CAD build for the part. Positions are in the model's coordinates, mm. Face numbers are marked on the shaded views. Give positions to 0.01 mm unless a question says otherwise; leave off trailing zeros. Write each loop counter-clockwise with the first axis right and the second up, starting at its lowest first coordinate (ties: lowest second). Pieces come first, ordered by that corner, then holes. Notation, with made-up numbers: (-30.5, -15.5) - (-0.5, -15.5) arc R27 cw to (-0.5, 2.5) - close; hole circle Ø2 at (31.25, 19). An arc over 180 degrees is marked (long way). Answer as a JSON object with one key per item and string values.
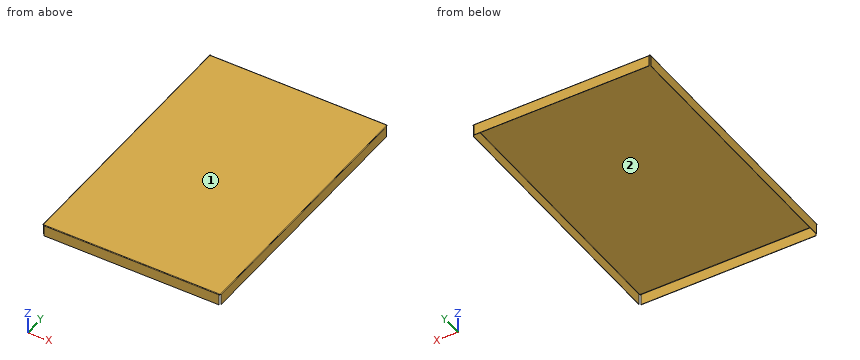
Autodesk Inventor part; units mm, degrees
ref_plane "YZ Plane" through (0, 0, 0) normal (1, 0, 0) x (0, 1, 0)
ref_plane "XZ Plane" through (0, 0, 0) normal (0, 1, 0) x (-1, 0, 0)
ref_plane "XY Plane" through (0, 0, 0) normal (0, 0, 1) x (1, 0, 0)
sketch "Boceto1" plane through (0, 0, 0) normal (0, 0, 1) x (1, 0, 0)
  line L0 (-19.05, -19.05) -> (-19.05, 19.05)
  line L1 (19.05, -19.05) -> (-19.05, -19.05)
  line L2 (-14.2875, 16.764) -> (-14.2875, -9.4615)
  line L3 (-9.4615, -14.2875) -> (16.764, -14.2875)
  arc A0 (-14.2875, -9.4615) -> (-9.4615, -14.2875) centre (-9.4615, -9.4615) ccw
  line L4 (-14.2875, -9.4615) -> (-14.2875, 871.3615)
  line L5 (-9.4615, 876.1875) -> (571.3615, 876.1875)
  line L6 (576.1875, 871.3615) -> (576.1875, -9.4615)
  line L7 (571.3615, -14.2875) -> (-9.4615, -14.2875)
  arc A1 (571.3615, -14.2875) -> (576.1875, -9.4615) centre (571.3615, -9.4615) ccw
  arc A2 (576.1875, 871.3615) -> (571.3615, 876.1875) centre (571.3615, 871.3615) ccw
  arc A3 (-9.4615, 876.1875) -> (-14.2875, 871.3615) centre (-9.4615, 871.3615) ccw
  line L8 (-14.2875, -9.4615) -> (-14.2875, -9.4615)
  arc A4 (-14.2875, -9.4615) -> (-9.4615, -14.2875) centre (-9.4615, -9.4615) ccw
  point P0 (0, 0)
  point P1 (-14.2875, -14.2875)
  point P2 (-14.2875, 876.1875)
  point P3 (576.1875, 876.1875)
  point P4 (576.1875, -14.2875)
  dimension "d3" = 890.475
  dimension "d5" = 890.475
  dimension "d6" = 4.826
  dimension "d7" = 4.826
  dimension "d8" = 4.826
  dimension "d9" = 4.826
sketch "Boceto1 outline for Placa1" plane through (0, 0, 0) normal (0, 0, 1) x (1, 0, 0)
  line L0 (-14.2875, -9.4615) -> (-14.2875, 871.3615)
  arc A0 (-14.2875, 871.3615) -> (-9.4615, 876.1875) centre (-9.4615, 871.3615) cw
  line L1 (-9.4615, 876.1875) -> (571.3615, 876.1875)
  arc A1 (571.3615, 876.1875) -> (576.1875, 871.3615) centre (571.3615, 871.3615) cw
  line L2 (576.1875, 871.3615) -> (576.1875, -9.4615)
  arc A2 (576.1875, -9.4615) -> (571.3615, -14.2875) centre (571.3615, -9.4615) cw
  line L3 (571.3615, -14.2875) -> (-9.4615, -14.2875)
  arc A3 (-9.4615, -14.2875) -> (-14.2875, -9.4615) centre (-9.4615, -9.4615) cw
extrude "Placa1" add sketch "Boceto1 outline for Placa1" along normal blind 1
sketch "Boceto2" plane through (-9.4615, -13.2875, 1) normal (0, -1, 0) x (1, 0, 0)
  line L0 (580.823, 0) -> (0, 0)
  line L1 (0, 0) -> (0, -38.1)
  line L2 (0, -38.1) -> (580.823, -38.1)
  line L3 (580.823, -38.1) -> (580.823, 0)
edge flange "Pestaña1" height 38.1 angle 90 thickness 1 bend radius 1 thickness toward (0, -1, 0) relief straight relief width 1 relief depth 0.5 corner gap 1 corner form 0 edges at (280.95, -14.2875, 0) (-14.2875, 430.95, 0) (280.95, 876.1875, 0) (576.1875, 430.95, 0) wall of the first edge with corners at (571.3615, -13.2875, 1) (-9.4615, -13.2875, 1) (-9.4615, -13.2875, -37.1) (571.3615, -13.2875, -37.1)
bend "Doblez1"
corner "Esquina1"
equation "\"d10\" = Anchura_desahogo_plegado"
equation "\"d11\" = Profundidad_desahogo_plegado"
equation "\"d12\" = Remanente_mínimo"
equation "\"d13\" = Radio_pliegue"
equation "\"d16\" = Radio_pliegue"
equation "\"d17\" = Tamaño_destalonado"
equation "\"d18\" = TamañoSeparación"
equation "\"d19\" = Tamaño_de_radio_de_Jacobi"
equation "\"Radio_pliegue\" = Grosor"
equation "\"Anchura_desahogo_plegado\" = Grosor"
equation "\"Profundidad_desahogo_plegado\" = 0.5 * Grosor"
equation "\"Tamaño_destalonado\" = 4 * Grosor"
equation "\"Remanente_mínimo\" = 2 * Grosor"
equation "\"Radiodetransición\" = Radio_pliegue"
equation "\"Tamaño_de_radio_de_Jacobi\" = Radio_pliegue"
equation "\"TamañoSeparación\" = Grosor"
equation "\"d2\" = Radio_pliegue"
properties part number "lámina" material "Latón, amarillo claro"
Item 1: Flat gauge pins, fed straight in: P1, Ø3, axis at y = -13.5, z = -24.5, coming from the +X side; P2, Ø2, axis at y = -13.5, z = -14, coming from the -X side; P3, Ø1.1, axis at y = -10, z = 0.5, coming from the +X side; P4, Ø0.8, axis at y = 874.5, z = -9, coming from the +X side. Where does each tip first touch, or does it go through?
Entries:
{"P1": "x = 571.36", "P2": "x = -9.46", "P3": "x = 576.08", "P4": "through"}
Item 2: Cut at B-B (y = 170). Give the cut face in (x, z), and give its area (3 significant figures).
Entries:
{"outline": "(-14.29, -37.1) - (-13.29, -37.1) - (-13.29, -1) arc R1 cw to (-12.29, 0) - (574.19, 0) arc R1 cw to (575.19, -1) - (575.19, -37.1) - (576.19, -37.1) - (576.19, -1) arc R2 ccw to (574.19, 1) - (-12.29, 1) arc R2 ccw to (-14.29, -1) - close", "area": "663 mm2"}
Item 3: Probe line 1 (X direction, y = 620.5, z = -33); line 2 (Y direction, x = 340, z = -20); line 3 (Z direction, x = 162, y = 499). List the from-to ranges inside material, lowest first. Write a range as from..to.
Entries:
{"line 1": "-14.29..-13.29, 575.19..576.19", "line 2": "-14.29..-13.29, 875.19..876.19", "line 3": "0..1"}
Item 4: Cut at C-C (x = 110). Give the cut face in (y, z), and give its area (3 significant figures).
Entries:
{"outline": "(-14.29, -37.1) - (-13.29, -37.1) - (-13.29, -1) arc R1 cw to (-12.29, 0) - (874.19, 0) arc R1 cw to (875.19, -1) - (875.19, -37.1) - (876.19, -37.1) - (876.19, -1) arc R2 ccw to (874.19, 1) - (-12.29, 1) arc R2 ccw to (-14.29, -1) - close", "area": "963 mm2"}
Item 5: Cut at A-A (z = -29.5). Give the cut face in (x, y).
Entries:
{"outline": "(-14.29, -9.46) - (-13.29, -9.46) - (-13.29, 871.36) - (-14.29, 871.36) - close; (-9.46, -14.29) - (571.36, -14.29) - (571.36, -13.29) - (-9.46, -13.29) - close; (-9.46, 875.19) - (571.36, 875.19) - (571.36, 876.19) - (-9.46, 876.19) - close; (575.19, -9.46) - (576.19, -9.46) - (576.19, 871.36) - (575.19, 871.36) - close"}
Item 6: Mould opens along Y. For the marked faces 1 and 2 say: +Y half, -Y half, draft (parallel to the pull), parting line (faces both ways), or undercut.
Entries:
{"face 1": "draft", "face 2": "undercut"}
